from build123d import *

# Parameters (mm, degrees)
SKETCH1_R         = 150
SKETCH1_R_2       = 97.5
SHROUD_DEPTH      = 3
SKETCH2_W         = 71.782300335
SKETCH2_H         = 3
BLADE_SLOTS_DEPTH = 3


with BuildPart() as part:
    # Sketch1 → Shroud (new body)
    with BuildSketch(Plane.XY):
        Circle(SKETCH1_R)
        Circle(SKETCH1_R_2, mode=Mode.SUBTRACT)
    extrude(amount=SHROUD_DEPTH)

    # Sketch2 → Blade_slots (cut)
    with BuildSketch(Plane.XY):
        with Locations((63.2155163, -96.418141453)):
            Rectangle(SKETCH2_W, SKETCH2_H)
        Polygon((83.872246927, -57.445884148), (138.860679213, -11.305110898), (136.932316384, -9.006977568), (81.943884098, -55.147750818), align=None)
        Polygon((101.175371248, 9.90594079), (113.64023689, 80.597706689), (110.685813631, 81.118651222), (98.220947989, 10.426885323), align=None)
        Polygon((71.137414923, 72.62266594), (35.246264756, 134.787961572), (32.648188544, 133.287961572), (68.539338712, 71.12266594), align=None)
        Polygon((7.813471551, 101.358438585), (-59.639826377, 125.909431234), (-60.665886807, 123.090353372), (6.787411121, 98.539360723), align=None)
        Polygon((-59.166481997, 82.667471343), (-126.619779924, 58.116478695), (-125.593719494, 55.297400832), (-58.140421567, 79.848393481), align=None)
        Polygon((-98.461781056, 25.295475513), (-134.352931224, -36.869820119), (-131.754855012, -38.369820119), (-95.863704845, 23.795475513), align=None)
        Polygon((-91.685718479, -43.912554438), (-79.220852837, -114.604320337), (-76.266429578, -114.083375804), (-88.73129522, -43.391609905), align=None)
        Polygon((-42.008889252, -92.573412133), (12.979543034, -138.714185383), (14.907905863, -136.416052054), (-40.080526423, -90.275278804), align=None)
    extrude(amount=BLADE_SLOTS_DEPTH, mode=Mode.SUBTRACT)


solid = part.part
Design review of the part built by this model. Coordinates are the model's own, in mm. A direction names the side the tool comes from. Round coordinates to 2 decimals unless told otherwise and drop trailing zeros. Write each loop counter-clockwise with the first axis right and the second up, starting at its lowest first coordinate (ties: lowest second). Pieces come first, ordered by that corner, then holes.
Item 1: Consider section D-D on z = 0.6. Count the separate pieces of the cut face and the enclosed holes in it, and give its area (3 significant figures).
Item 2: For pin 1 Ø1 at (y, z) = (21, 1) entering from -X; pin 2 Ø0.9 at (x, z) = (47, 1) entering from -Y; pin 3 Ø0.9 at (y, z) = (-96, 2) entering from +X, all flat-tipped, find the tip position at first contact; note any pin that passes through.
Item 3: Consider section B-B on y = -4. Give the boundary of the cut face in (x, z), and give its area (3 significant figures).
Item 4: Consider section A-A on x = -33. Give the boundary of the cut face in (y, z), and give its area (3 significant figures).
Item 5: Consider section C-C on x = -116. Give the boundary of the cut face in (y, z).
Item 6: Draft analysis for pull direction X (two halves, no side actions). For faces 1 (the cylindrical face through (-77.37, -59.33, 1.48)), 2 (the cylindrical face through (-19.527, 148.724, 1.479)), 3 (the flat face through (98, 2, 0)), state which applies: released by +X, released by -X, zero draft, split by the parting line, or undercut.
Item 7: Wall thickness on L1, parallel to X at y = 15, z = 1.5; L2, parallel to X at y = 45, z = 2.6; L3, parallel to Y at x = 65, z = 0.2: over which ranges is each line inside the solid? List them lowest first.
Item 8: For faces 4 (the flat face through (98, 2, 3)), 5 (the flat face through (-12.2, -113.67, 1.48)), list the 3-axis set-ups (+Z, -Z, +X, -X, +Y, -Y) from which the entire face can be reached by the end or side of a thin tool; tool diameter is ignored.
Check values:
1. separate pieces: 1
1. enclosed holes: 10
1. area: 38,900 mm2
2. pin 1: stops at x = -148.59
2. pin 2: stops at y = -142.59
2. pin 3: stops at x = 115.63
3. outline: (-149.95, 0) - (-115.38, 0) - (-115.38, 3) - (-149.95, 3) - close; (-111.91, 0) - (-97.42, 0) - (-97.42, 3) - (-111.91, 3) - close; (97.42, 0) - (149.95, 0) - (149.95, 3) - (97.42, 3) - close
3. area: 305 mm2
4. outline: (-146.32, 0) - (-100.13, 0) - (-100.13, 3) - (-146.32, 3) - close; (-96.22, 0) - (-91.75, 0) - (-91.75, 3) - (-96.22, 3) - close; (91.75, 0) - (113.02, 0) - (113.02, 3) - (91.75, 3) - close; (116.21, 0) - (146.32, 0) - (146.32, 3) - (116.21, 3) - close
4. area: 306 mm2
5. outline: (-95.1, 0) - (-11.08, 0) - (-11.08, 3) - (-95.1, 3) - close; (-5.08, 0) - (58.79, 0) - (58.79, 3) - (-5.08, 3) - close; (61.98, 0) - (95.1, 0) - (95.1, 3) - (61.98, 3) - close
6. face 1: undercut
6. face 2: split by the parting line
6. face 3: zero draft
7. L1: x = -149.25 to -104.41, -100.94 to -96.34, 96.34 to 99.03, 102.07 to 149.25
7. L2: x = -143.09 to -86.49, 86.49 to 104.32, 107.36 to 143.09
7. L3: y = -135.19 to -97.92, -94.92 to -72.67, 72.67 to 77.25, 83.25 to 135.19
8. face 4: +Z, +X, -X, +Y, -Y
8. face 5: +Z, -Z
